from build123d import *

# Parameters (mm, degrees)
SKETCH1_R             = 15
SKETCH1_R_2           = 12
BOSS_EXTRUDE1_DEPTH   = 85
CHAMFER1_SIZE         = 1
SKETCH2_R             = 12
SKETCH2_R_2           = 10
BOSS_EXTRUDE2_DEPTH   = 5
CUT_EXTRUDE1_DEPTH    = 3
CIRPATTERN1_COUNT     = 12
MIRROR2_COPY_1_DEPTH  = 3
MIRROR2_COPY_2_DEPTH  = 3
MIRROR2_COPY_3_DEPTH  = 3
MIRROR2_COPY_4_DEPTH  = 3
MIRROR2_COPY_5_DEPTH  = 3
MIRROR2_COPY_6_DEPTH  = 3
MIRROR2_COPY_7_DEPTH  = 3
MIRROR2_COPY_8_DEPTH  = 3
MIRROR2_COPY_9_DEPTH  = 3
MIRROR2_COPY_10_DEPTH = 3
MIRROR2_COPY_11_DEPTH = 3


with BuildPart() as part:
    # Sketch1 → Boss-Extrude1 (new, symmetric)
    with BuildSketch(Plane.XY):
        Circle(SKETCH1_R)
        Circle(SKETCH1_R_2, mode=Mode.SUBTRACT)
    extrude(amount=BOSS_EXTRUDE1_DEPTH, both=True)

    # Chamfer1
    chamfer1_edges = [part.edges().sort_by_distance(p)[0] for p in [
        (-15, 0, -85),
        (-15, 0, 85),
    ]]
    chamfer(chamfer1_edges, length=CHAMFER1_SIZE)

    # Sketch2 → Boss-Extrude2 (add)
    with BuildSketch(Plane(origin=(0, 0, -85), x_dir=(-1, 0, 0), z_dir=(0, 0, -1))):
        Circle(SKETCH2_R)
        Circle(SKETCH2_R_2, mode=Mode.SUBTRACT)
    boss_extrude2 = extrude(amount=-BOSS_EXTRUDE2_DEPTH)

    # Mirror1: Boss-Extrude2 across plane
    add(boss_extrude2.mirror(Plane.XY))

    # Sketch3 → Cut-Extrude1 (cut)
    with BuildSketch(Plane(origin=(0, 0, -85), x_dir=(-1, 0, 0), z_dir=(0, 0, -1))):
        with BuildLine():
            Line((-1.435788114, 10.905893475), (-1.762103595, 13.384505629))
            ThreePointArc((-1.762103595, 13.384505629), (0, 13.5), (1.762103595, 13.384505629))
            Line((1.762103595, 13.384505629), (1.435788114, 10.905893475))
            ThreePointArc((1.435788114, 10.905893475), (0, 11), (-1.435788114, 10.905893475))
        make_face()
    cut_extrude1 = extrude(amount=-CUT_EXTRUDE1_DEPTH, mode=Mode.SUBTRACT)

    # CirPattern1: Cut-Extrude1 ×12 about axis
    cirpattern1_axis = Axis((0, 0, 0), (0, 0, 1))
    for i in range(1, CIRPATTERN1_COUNT):
        add(cut_extrude1.rotate(cirpattern1_axis, i * 360 / CIRPATTERN1_COUNT), mode=Mode.SUBTRACT)

    # Mirror2: Cut-Extrude1 across plane
    add(cut_extrude1.mirror(Plane.XY), mode=Mode.SUBTRACT)

    # Mirror2 copy 1 sketch → Mirror2 copy 1 (cut)
    with BuildSketch(Plane(origin=(0, 0, 85), x_dir=(-0.8660254037844387, -0.49999999999999994, 0), z_dir=(0, 0, 1))):
        with BuildLine():
            Line((-1.435788114, -10.905893475), (-1.762103595, -13.384505629))
            ThreePointArc((-1.762103595, -13.384505629), (0, -13.5), (1.762103595, -13.384505629))
            Line((1.762103595, -13.384505629), (1.435788114, -10.905893475))
            ThreePointArc((1.435788114, -10.905893475), (0, -11), (-1.435788114, -10.905893475))
        make_face()
    extrude(amount=-MIRROR2_COPY_1_DEPTH, mode=Mode.SUBTRACT)

    # Mirror2 copy 2 sketch → Mirror2 copy 2 (cut)
    with BuildSketch(Plane(origin=(0, 0, 85), x_dir=(-0.5000000000000001, -0.8660254037844386, 0), z_dir=(0, 0, 1))):
        with BuildLine():
            Line((-1.435788114, -10.905893475), (-1.762103595, -13.384505629))
            ThreePointArc((-1.762103595, -13.384505629), (0, -13.5), (1.762103595, -13.384505629))
            Line((1.762103595, -13.384505629), (1.435788114, -10.905893475))
            ThreePointArc((1.435788114, -10.905893475), (0, -11), (-1.435788114, -10.905893475))
        make_face()
    extrude(amount=-MIRROR2_COPY_2_DEPTH, mode=Mode.SUBTRACT)

    # Mirror2 copy 3 sketch → Mirror2 copy 3 (cut)
    with BuildSketch(Plane(origin=(0, 0, 85), x_dir=(0, -1, 0), z_dir=(0, 0, 1))):
        with BuildLine():
            Line((-1.435788114, -10.905893475), (-1.762103595, -13.384505629))
            ThreePointArc((-1.762103595, -13.384505629), (0, -13.5), (1.762103595, -13.384505629))
            Line((1.762103595, -13.384505629), (1.435788114, -10.905893475))
            ThreePointArc((1.435788114, -10.905893475), (0, -11), (-1.435788114, -10.905893475))
        make_face()
    extrude(amount=-MIRROR2_COPY_3_DEPTH, mode=Mode.SUBTRACT)

    # Mirror2 copy 4 sketch → Mirror2 copy 4 (cut)
    with BuildSketch(Plane(origin=(0, 0, 85), x_dir=(0.4999999999999998, -0.8660254037844387, 0), z_dir=(0, 0, 1))):
        with BuildLine():
            Line((-1.435788114, -10.905893475), (-1.762103595, -13.384505629))
            ThreePointArc((-1.762103595, -13.384505629), (0, -13.5), (1.762103595, -13.384505629))
            Line((1.762103595, -13.384505629), (1.435788114, -10.905893475))
            ThreePointArc((1.435788114, -10.905893475), (0, -11), (-1.435788114, -10.905893475))
        make_face()
    extrude(amount=-MIRROR2_COPY_4_DEPTH, mode=Mode.SUBTRACT)

    # Mirror2 copy 5 sketch → Mirror2 copy 5 (cut)
    with BuildSketch(Plane(origin=(0, 0, 85), x_dir=(0.8660254037844387, -0.49999999999999994, 0), z_dir=(0, 0, 1))):
        with BuildLine():
            Line((-1.435788114, -10.905893475), (-1.762103595, -13.384505629))
            ThreePointArc((-1.762103595, -13.384505629), (0, -13.5), (1.762103595, -13.384505629))
            Line((1.762103595, -13.384505629), (1.435788114, -10.905893475))
            ThreePointArc((1.435788114, -10.905893475), (0, -11), (-1.435788114, -10.905893475))
        make_face()
    extrude(amount=-MIRROR2_COPY_5_DEPTH, mode=Mode.SUBTRACT)

    # Mirror2 copy 6 sketch → Mirror2 copy 6 (cut)
    with BuildSketch(Plane.XY.offset(85)):
        with BuildLine():
            Line((-1.435788114, -10.905893475), (-1.762103595, -13.384505629))
            ThreePointArc((-1.762103595, -13.384505629), (0, -13.5), (1.762103595, -13.384505629))
            Line((1.762103595, -13.384505629), (1.435788114, -10.905893475))
            ThreePointArc((1.435788114, -10.905893475), (0, -11), (-1.435788114, -10.905893475))
        make_face()
    extrude(amount=-MIRROR2_COPY_6_DEPTH, mode=Mode.SUBTRACT)

    # Mirror2 copy 7 sketch → Mirror2 copy 7 (cut)
    with BuildSketch(Plane(origin=(0, 0, 85), x_dir=(0.8660254037844386, 0.5000000000000001, 0), z_dir=(0, 0, 1))):
        with BuildLine():
            Line((-1.435788114, -10.905893475), (-1.762103595, -13.384505629))
            ThreePointArc((-1.762103595, -13.384505629), (0, -13.5), (1.762103595, -13.384505629))
            Line((1.762103595, -13.384505629), (1.435788114, -10.905893475))
            ThreePointArc((1.435788114, -10.905893475), (0, -11), (-1.435788114, -10.905893475))
        make_face()
    extrude(amount=-MIRROR2_COPY_7_DEPTH, mode=Mode.SUBTRACT)

    # Mirror2 copy 8 sketch → Mirror2 copy 8 (cut)
    with BuildSketch(Plane(origin=(0, 0, 85), x_dir=(0.5000000000000004, 0.8660254037844384, 0), z_dir=(0, 0, 1))):
        with BuildLine():
            Line((-1.435788114, -10.905893475), (-1.762103595, -13.384505629))
            ThreePointArc((-1.762103595, -13.384505629), (0, -13.5), (1.762103595, -13.384505629))
            Line((1.762103595, -13.384505629), (1.435788114, -10.905893475))
            ThreePointArc((1.435788114, -10.905893475), (0, -11), (-1.435788114, -10.905893475))
        make_face()
    extrude(amount=-MIRROR2_COPY_8_DEPTH, mode=Mode.SUBTRACT)

    # Mirror2 copy 9 sketch → Mirror2 copy 9 (cut)
    with BuildSketch(Plane(origin=(0, 0, 85), x_dir=(0, 1, 0), z_dir=(0, 0, 1))):
        with BuildLine():
            Line((-1.435788114, -10.905893475), (-1.762103595, -13.384505629))
            ThreePointArc((-1.762103595, -13.384505629), (0, -13.5), (1.762103595, -13.384505629))
            Line((1.762103595, -13.384505629), (1.435788114, -10.905893475))
            ThreePointArc((1.435788114, -10.905893475), (0, -11), (-1.435788114, -10.905893475))
        make_face()
    extrude(amount=-MIRROR2_COPY_9_DEPTH, mode=Mode.SUBTRACT)

    # Mirror2 copy 10 sketch → Mirror2 copy 10 (cut)
    with BuildSketch(Plane(origin=(0, 0, 85), x_dir=(-0.5000000000000001, 0.8660254037844386, 0), z_dir=(0, 0, 1))):
        with BuildLine():
            Line((-1.435788114, -10.905893475), (-1.762103595, -13.384505629))
            ThreePointArc((-1.762103595, -13.384505629), (0, -13.5), (1.762103595, -13.384505629))
            Line((1.762103595, -13.384505629), (1.435788114, -10.905893475))
            ThreePointArc((1.435788114, -10.905893475), (0, -11), (-1.435788114, -10.905893475))
        make_face()
    extrude(amount=-MIRROR2_COPY_10_DEPTH, mode=Mode.SUBTRACT)

    # Mirror2 copy 11 sketch → Mirror2 copy 11 (cut)
    with BuildSketch(Plane(origin=(0, 0, 85), x_dir=(-0.8660254037844384, 0.5000000000000004, 0), z_dir=(0, 0, 1))):
        with BuildLine():
            Line((-1.435788114, -10.905893475), (-1.762103595, -13.384505629))
            ThreePointArc((-1.762103595, -13.384505629), (0, -13.5), (1.762103595, -13.384505629))
            Line((1.762103595, -13.384505629), (1.435788114, -10.905893475))
            ThreePointArc((1.435788114, -10.905893475), (0, -11), (-1.435788114, -10.905893475))
        make_face()
    extrude(amount=-MIRROR2_COPY_11_DEPTH, mode=Mode.SUBTRACT)


solid = part.part
The listing builds one solid part. Answer for the finished solid, in the listing's coordinates (mm). A direction names the side the tool comes from. Give positions to 0.01 mm unless a question says otherwise; leave off trailing zeros. Loops run counter-clockwise (first coordinate to the right, second up) from the corner with the lowest first, then second, coordinate; pieces in that order, holes last. Notation, with made-up numbers: (86.5, -17) - (109.5, -17) arc R30 cw to (109.5, 6) - close; hole circle Ø1 at (-18, 27). An arc over 180 degrees is marked (long way). Use one line per item in the form item = value.
1. Given pin 1 Ø1.1 at (x, y) = (-5, -10.5) entering from -Z; pin 2 Ø6 at (y, z) = (10, 25.5) entering from +X; pin 3 Ø5 at (x, y) = (4.5, 5.5) entering from -Z; pin 4 Ø1 at (y, z) = (7, 30) entering from -X, each flat-ended and moving along its own axis, determine where each tip first touches the part or whether it passes through.
Calculated:
pin_1 = -82
pin_2 = 13.27
pin_3 = through
pin_4 = -13.52
2. Section A-A on z = 13.5 is taken. Give the vertices of the cut face in (x, y).
Calculated:
outline = circle Ø30 at (0, 0); hole circle Ø24 at (0, 0)
3. The mould has two halves that part along X. Classify faces 4 (the face through (-11.704, -6.729, 83.521)), 5 (the face through (-14.985, 0.66, 1.176)): pulls with the +X half, pulls with the -X half, needs draft (parallel to the pull), parting line crosses it, or undercut.
Calculated:
face_4 = undercut
face_5 = parting line crosses it
4. Which of the six approach directions +Z, -Z, +X, -X, +Y, -Y give full straight-line access (tool end or side, diameter ignored) to faces 1 (the face through (5, 9, 80)), 2 (the face through (-6.77, -11.68, 83.52)), 3 (the face through (11, 0, -84))?
Calculated:
face_1 = none
face_2 = +Z
face_3 = -Z
5. Find the intervals of material crossed by line 1 along Y through (x, z) = (0, -82.1); line 2 along Z through (x, y) = (-3.25, 10.5); line 3 along Y through (x, z) = (0, 1.5), in increasing order. Write a range as [from, to].
Calculated:
line_1 = [-15, -13.5], [-11, -10], [10, 11], [13.5, 15]
line_2 = [-85, -80], [80, 85]
line_3 = [-15, -12], [12, 15]
